Input: part model. Units: mm. Frame: model coordinates. A direction names the side the tool comes from. Give positions to 0.01 mm unless a question says otherwise; leave off trailing zeros. Write each loop counter-clockwise with the first axis right and the second up, starting at its lowest first coordinate (ties: lowest second). Pieces come first, ordered by that corner, then holes. Notation, with made-up numbers: (6.25, -37) - (50.25, -37) arc R33 ccw to (50.25, -4) - close; hole circle Ø3 at (-14.5, 2.5). An arc over 180 degrees is marked (long way). Use a Markdown table: item, result. Add a question column.
1. Section query A-A, the plane z = 1.3. Return loops of the section in (x, y).
2. Set-up query: faces 4 (the flat face through (-54, 36, 3.5)), 5 (the flat face through (-54, 36, 5)), 6 (the cylindrical face through (-51.95, 36.5, 4.14)). Return all of +Z, -Z, +X, -X, +Y, -Y with unobstructed straight access to the full face (end or side cutting, diameter ignored); none if empty.
3. Pin query (flat end, axial travel): pin 1 (1.6 mm diameter, centred on x = -50.33, y = 35.75, fed in from +Z); pin 2 (2.5 mm diameter, centred on x = -54.33, y = 35.75, fed in from -Z). Return the tip coordinate at first contact, or that it passes through.
4. Mould query, pull axis X, two halves, no side actions, for faces 1 (the flat face through (-50, 33, 0)), 2 (the cylindrical face through (-55, 35, 3)), 3 (the flat face through (-42.334, 36, 2)). Classes: released by +X, released by -X, zero draft, split by the parting line, or undercut.
5. Material intervals for probe 1 along Y at (x, z) = (-52.75, 1.45); probe 2 along X at (y, z) = (36.25, 3.4); probe 3 along Z at (x, y) = (-55.25, 38.5), sorted ascending.
6. Section query C-C, the plane z = 2.85. Return loops of the section in (x, y).
7. Section query D-D, the plane x = -54.25. Return loops of the section in (y, z), plus the area to 3 significant figures.
```python
from build123d import *

# Parameters (mm, degrees)
F0_W        = 16
F0_H        = 8
F1_DEPTH    = 3.3
F3_R        = 2.5
F4_DEPTH    = 1.7
F6_T        = -1.5
F7_DEPTH    = 3.3
F8_T        = 0.8
F8_T3_DEPTH = 3.4
F8_T5_DEPTH = 6.6
F8_T7_DEPTH = 14.6


# Not quite as in the source:
# - a shell that OpenCascade refuses in one call is made with other operations: the cavity is built on its own and cut out


with BuildPart() as f1:
    # F0 (on Top) → F1 (new body)
    with BuildSketch(Plane.XY):
        with Locations((-50.3335684606, 35.747165516)):
            Rectangle(F0_W, F0_H)
    extrude(amount=F1_DEPTH)

    # F3 (on face) → F4 (join)
    with BuildSketch(Plane.XY.offset(3.3)):
        with Locations((-46.3335684606, 35.747165516)):
            Circle(F3_R)
        with Locations((-54.3335684606, 35.747165516)):
            Circle(F3_R)
    extrude(amount=F4_DEPTH)

    # F6
    f6_openings = [f1.faces().sort_by_distance(p)[0] for p in [
        (-50.333568, 35.747166, 0),
    ]]
    offset(amount=F6_T, openings=f6_openings, kind=Kind.INTERSECTION)

    # F5 (on face) → F7 (join)
    with BuildSketch(Plane.XY.offset(3.3)):
        with BuildLine():
            ThreePointArc((-51.8335684606, 35.747165516), (-50.3335684606, 34.247165516), (-48.8335684606, 35.747165516))
            ThreePointArc((-48.8335684606, 35.747165516), (-50.3335684606, 37.247165516), (-51.8335684606, 35.747165516))
        make_face()
    extrude(amount=-F7_DEPTH)

    # F8: shell of thickness 0.8, made by hand


with BuildPart() as f8_core1:
    # F8_t2: copy of F1
    add(f1.part)

    # the walls: a layer under each face that stays
    f8_faces = [f8_core1.faces().sort_by_distance(p)[0] for p in [
        (-50.3335684606, 39.747165516, 1.65),
        (-50.3335684606, 35.747165516, 3.3),
        (-48.8335684606, 35.747165516, 4.15),
        (-46.3335684606, 35.747165516, 5),
        (-56.8335684606, 35.747165516, 4.15),
        (-54.3335684606, 35.747165516, 5),
        (-50.3335684606, 31.747165516, 1.65),
        (-55.666901794, 33.0804988494, 0),
        (-56.8335684606, 35.747165516, 0.9),
        (-54.666901794, 34.0804988494, 1.8),
        (-47.3335684606, 35.747165516, 2.65),
        (-46.3335684606, 35.747165516, 3.5),
        (-48.8335684606, 35.747165516, 0.9),
        (-55.3335684606, 35.747165516, 2.65),
        (-54.3335684606, 35.747165516, 3.5),
        (-50.3335684606, 33.247165516, 0.9),
        (-43.8335684606, 35.747165516, 0.9),
        (-50.3335684606, 38.247165516, 0.9),
        (-58.3335684606, 35.747165516, 1.65),
        (-42.3335684606, 35.747165516, 1.65),
    ]]
    thicken(f8_faces, amount=-F8_T, mode=Mode.SUBTRACT)

    # F8_s4 → F8_t3 (cut)
    with BuildSketch(Plane.XY.offset(-0.8)):
        Polygon((-56.8255684606, 33.255165516), (-57.6335684606, 33.247165516), (-57.6335684606, 32.447165516), (-56.8335684606, 32.447165516), align=None)
        Polygon((-56.8255684606, 38.239165516), (-57.6335684606, 38.247165516), (-57.6335684606, 39.047165516), (-56.8335684606, 39.047165516), align=None)
        Polygon((-43.8415684606, 33.255165516), (-43.8335684606, 32.447165516), (-43.0335684606, 32.447165516), (-43.0335684606, 33.247165516), align=None)
        Polygon((-43.8415684606, 38.239165516), (-43.0335684606, 38.247165516), (-43.0335684606, 39.047165516), (-43.8335684606, 39.047165516), align=None)
    extrude(amount=F8_T3_DEPTH, mode=Mode.SUBTRACT)

    # F8_s6 → F8_t5 (cut)
    with BuildSketch(Plane.XZ.offset(-39.047165516)):
        Polygon((-56.8255684606, 1.792), (-57.6335684606, 1.8), (-57.6335684606, 2.6), (-56.8335684606, 2.6), align=None)
        Polygon((-43.8415684606, 1.792), (-43.8335684606, 2.6), (-43.0335684606, 2.6), (-43.0335684606, 1.8), align=None)
    extrude(amount=F8_T5_DEPTH, mode=Mode.SUBTRACT)

    # F8_s8 → F8_t7 (cut)
    with BuildSketch(Plane.YZ.offset(-57.6335684606)):
        Polygon((33.255165516, 1.792), (33.247165516, 2.6), (32.447165516, 2.6), (32.447165516, 1.8), align=None)
        Polygon((38.239165516, 1.792), (38.247165516, 2.6), (39.047165516, 2.6), (39.047165516, 1.8), align=None)
    extrude(amount=F8_T7_DEPTH, mode=Mode.SUBTRACT)

    # F8_s9 → F8_t10 (revolve, cut)
    with BuildSketch(Plane.XZ.offset(-35.747165516)):
        Polygon((-51.8255684606, 3.308), (-51.8335684606, 2.5), (-52.6335684606, 2.5), (-52.6335684606, 3.3), align=None)
    revolve(axis=Axis((-54.3335684606, 35.747165516, 3.3), (0, 0, 1)), mode=Mode.SUBTRACT)

    # F8_s11 → F8_t12 (revolve, cut)
    with BuildSketch(Plane.XZ.offset(-35.747165516)):
        Polygon((-43.8255684606, 3.308), (-43.8335684606, 2.5), (-44.6335684606, 2.5), (-44.6335684606, 3.3), align=None)
    revolve(axis=Axis((-46.3335684606, 35.747165516, 3.3), (0, 0, -1)), mode=Mode.SUBTRACT)

    # F8_s13 → F8_t14 (revolve, cut)
    with BuildSketch(Plane.XZ.offset(-35.747165516)):
        Polygon((-51.8415684606, 1.792), (-51.8335684606, 2.6), (-51.0335684606, 2.6), (-51.0335684606, 1.8), align=None)
    revolve(axis=Axis((-50.3335684606, 35.747165516, 1.8), (0, 0, 1)), mode=Mode.SUBTRACT)

    # F8_s15 → F8_t16 (revolve, cut)
    with BuildSketch(Plane.XZ.offset(-35.747165516)):
        Polygon((-45.3415684606, 3.492), (-44.5335684606, 3.5), (-44.5335684606, 4.3), (-45.3335684606, 4.3), align=None)
    revolve(axis=Axis((-46.3335684606, 35.747165516, 3.5), (0, 0, -1)), mode=Mode.SUBTRACT)

    # F8_s17 → F8_t18 (revolve, cut)
    with BuildSketch(Plane.XZ.offset(-35.747165516)):
        Polygon((-53.3415684606, 3.492), (-52.5335684606, 3.5), (-52.5335684606, 4.3), (-53.3335684606, 4.3), align=None)
    revolve(axis=Axis((-54.3335684606, 35.747165516, 3.5), (0, 0, -1)), mode=Mode.SUBTRACT)


with BuildPart() as f1_1:
    add(f1.part)

    # what is left inside the walls is the cavity
    f8_cavity = [f8_core1.part.solids().sort_by_distance(p)[0] for p in [
        (-49.641568, 35.747166, 1.666667),
    ]]
    add(f8_cavity, mode=Mode.SUBTRACT)


solid = f1_1.part
```
Result sheet:
| question | item | result |
|---|---|---|
| 1 | outline | (-58.33, 31.75) - (-42.33, 31.75) - (-42.33, 39.75) - (-58.33, 39.75) - close; circle Ø3 at (-50.33, 35.75); hole (-56.83, 33.25) - (-43.83, 33.25) - (-43.83, 38.25) - (-56.83, 38.25) - close; hole circle Ø1.4 at (-50.33, 35.75) |
| 2 | face 4 | -Z |
| 2 | face 5 | +Z, +X, -X, +Y, -Y |
| 2 | face 6 | +Z |
| 3 | pin 1 | stops at z = 3.3 |
| 3 | pin 2 | stops at z = 1.8 |
| 4 | face 1 | zero draft |
| 4 | face 2 | undercut |
| 4 | face 3 | released by +X |
| 5 | probe 1 | y = 31.75 to 33.25, 38.25 to 39.75 |
| 5 | probe 2 | x = -56.78 to -55.2, -53.47 to -51.88, -48.78 to -47.2, -45.47 to -43.88 |
| 5 | probe 3 | z = 0 to 3.3 |
| 6 | outline | (-58.33, 31.75) - (-42.33, 31.75) - (-42.33, 39.75) - (-58.33, 39.75) - close; hole circle Ø2 at (-54.33, 35.75); hole circle Ø2 at (-46.33, 35.75) |
| 7 | outline | (31.75, 0) - (33.25, 0) - (33.25, 1.8) - (34.75, 1.8) - (34.75, 3.5) - (36.74, 3.5) - (36.74, 1.8) - (38.25, 1.8) - (38.25, 0) - (39.75, 0) - (39.75, 3.3) - (38.25, 3.3) - (38.25, 5) - (33.25, 5) - (33.25, 3.3) - (31.75, 3.3) - close |
| 7 | area | 22.5 mm² |
